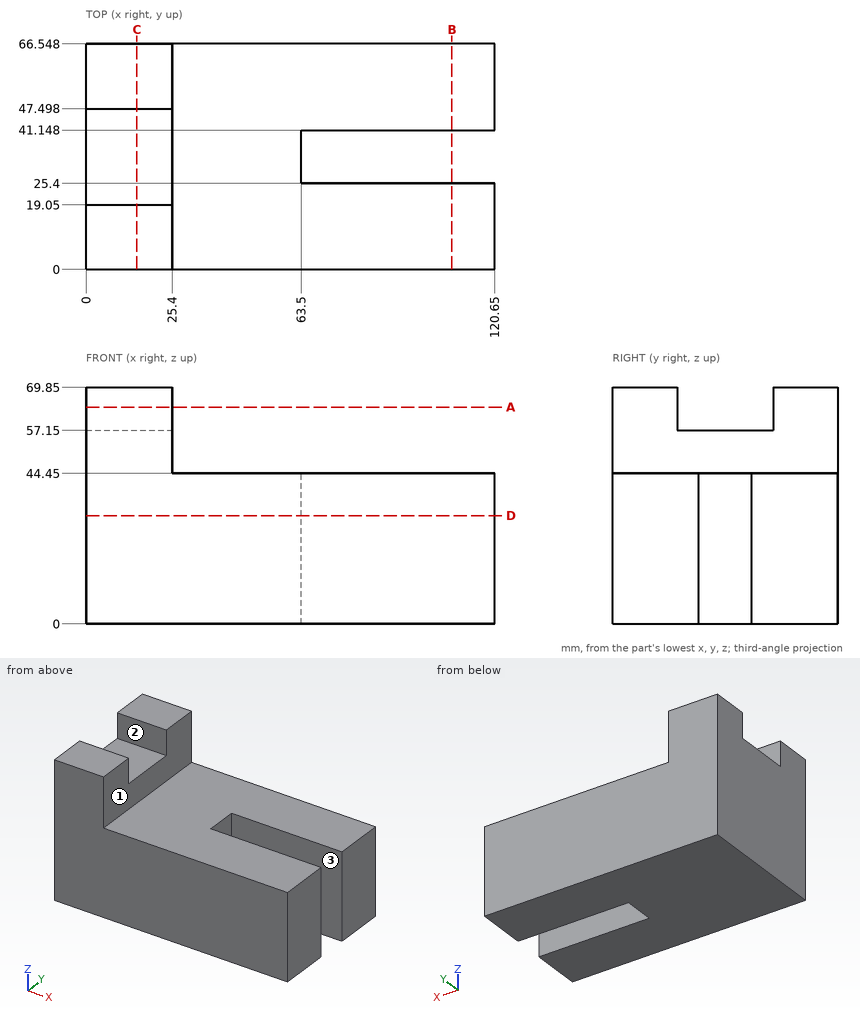
For this review, use the dimensioned drawing (mm, ordinates from the lowest corner) and the shaded views. A direction names the side the tool comes from. Round coordinates to 2 decimals unless told otherwise and drop trailing zeros. Write each loop counter-clockwise with the first axis right and the second up, starting at its lowest first coordinate (ties: lowest second). Pieces come first, ordered by that corner, then holes. Notation, with made-up numbers: (50.25, -33) -> (85.25, -33) arc R8 ccw to (85.25, -27) -> close; hole circle Ø8 at (68, 45.5). An arc over 180 degrees is marked (long way). One line per item, written item: value. Start each with the question number.
Q1. Add section D-D (z = 32). Give the boundary of the cut face in (x, y), then the cut area to 3 significant figures.
Q2. Insertion check: P1, Ø8, axis at y = 31, z = 17.5, coming from the +X side. The pin has a flat end and moves straight along its axis. Give the tip position at first contact, or say it passes through.
Q3. To check wall thickness, follow probe 1 along Y at (x, z) = (98, 7); probe 2 along Z at (x, y) = (34, 38); probe 3 along X at (y, z) = (63, 46.5). State the ranges of each line that lie inside material, in increasing order.
Q4. Add section B-B (x = 108). Give the boundary of the cut face in (y, z), then the cut area to 3 significant figures.
Q5. Add section C-C (x = 15). Give the boundary of the cut face in (y, z).
Q6. Tool access review of the marked faces 1, 2 and 3: name each direction out of +Z, -Z, +X, -X, +Y, -Y from which nothing blocks a thin tool from reaching the whole face with its end or side.
Q7. Add section A-A (z = 64). Give the boundary of the cut face in (x, y).
Response:
1. outline: (0, 0) -> (120.65, 0) -> (120.65, 25.4) -> (63.5, 25.4) -> (63.5, 41.15) -> (120.65, 41.15) -> (120.65, 66.55) -> (0, 66.55) -> close
1. area: 7,130 mm^2
2. P1: stops at x = 63.5
3. probe 1: y = 0 to 25.4, 41.15 to 66.55
3. probe 2: z = 0 to 44.45
3. probe 3: x = 0 to 25.4
4. outline: (0, 0) -> (25.4, 0) -> (25.4, 44.45) -> (0, 44.45) -> close; (41.15, 0) -> (66.55, 0) -> (66.55, 44.45) -> (41.15, 44.45) -> close
4. area: 2,260 mm^2
5. outline: (0, 0) -> (66.55, 0) -> (66.55, 69.85) -> (47.5, 69.85) -> (47.5, 57.15) -> (19.05, 57.15) -> (19.05, 69.85) -> (0, 69.85) -> close
6. face 1: +Z, +X, +Y, -Y
6. face 2: +Z, +X, -X
6. face 3: +Z, -Z, +X
7. outline: (0, 0) -> (25.4, 0) -> (25.4, 19.05) -> (0, 19.05) -> close; (0, 47.5) -> (25.4, 47.5) -> (25.4, 66.55) -> (0, 66.55) -> close
